Input: part model. Units: mm. Frame: model coordinates. Face numbers are marked on the shaded views. Give positions to 0.01 mm unless a question says otherwise; leave off trailing zeros. Loops run counter-clockwise (first coordinate to the right, second up) from the corner with the lowest first, then second, coordinate; pieces in that order, holes last. Notation, with made-up numbers: (52, 33) -> (56, 33) arc R29 cw to (56, 68) -> close; hole circle Ø9 at (72, 27). An arc over 180 degrees is marked (long way). Use CSV: the item, a comma, the result in double quotes.
```python
from build123d import *
from OCP.BRepFilletAPI import BRepFilletAPI_MakeChamfer

# Parameters (mm, degrees)
BOSS_EXTRUDE1_DEPTH  = 13.335
SKETCH2_R            = 13.97
BOSS_EXTRUDE2_DEPTH  = 2.54
BOSS_EXTRUDE3_DEPTH  = 36.068
BOSS_EXTRUDE4_START  = 6.477
SKETCH3_R            = 10.287
BOSS_EXTRUDE4_DEPTH  = 3.937
CHAMFER1_SIZE        = 0.254
CHAMFER1_EDGE_2_SIZE = 0.254
CHAMFER1_EDGE_3_SIZE = 0.254
CHAMFER1_EDGE_4_SIZE = 0.254
CHAMFER1_EDGE_5_SIZE = 0.254
CHAMFER1_EDGE_6_SIZE = 0.254
SKETCH4_W            = 12.192
SKETCH4_H            = 7.3025
CUT_EXTRUDE1_DEPTH   = 10.922
SKETCH5_W            = 6.35
SKETCH5_H            = 2.54
CUT_EXTRUDE2_DEPTH   = 6.35
SKETCH6_R            = 13.267076916
BOSS_EXTRUDE5_DEPTH  = 1.27
BOSS_EXTRUDE6_DEPTH  = 1.27
SKETCH8_R            = 2.54
BOSS_EXTRUDE7_DEPTH  = 2.54
FILLET1_R            = 1.27
SKETCH9_R            = 11.938
BOSS_EXTRUDE8_DEPTH  = 12.065
SKETCH10_R           = 13.97
BOSS_EXTRUDE9_DEPTH  = 2.54
SKETCH11_R           = 10.287
CUT_EXTRUDE3_DEPTH   = 6.223
SKETCH12_R           = 1.27
BOSS_EXTRUDE10_DEPTH = 9.525
CIRPATTERN1_COUNT    = 10
CHAMFER2_SIZE        = 1.27
CHAMFER2_SIZE2       = 0.733234842


with BuildPart() as part:
    # Sketch1 → Boss-Extrude1 (new body)
    with BuildSketch(Plane(origin=(0, 0, 0), x_dir=(1, 0, 0), z_dir=(0, 1, 0))):
        with BuildLine():
            Line((8.7122, -5.469912263), (8.7122, 5.469912263))
            ThreePointArc((8.7122, 5.469912263), (-10.287, 0), (8.7122, -5.469912263))
        make_face()
    extrude(amount=BOSS_EXTRUDE1_DEPTH)

    # Sketch2 → Boss-Extrude2 (add)
    with BuildSketch(Plane(origin=(0, 13.335, 0), x_dir=(1, 0, 0), z_dir=(0, 1, 0))):
        with Locations(Location((0, 0, 0), (0, 0, 270))):
            Circle(SKETCH2_R)
    extrude(amount=BOSS_EXTRUDE2_DEPTH)

    # Sketch1<2> → Boss-Extrude3 (add)
    with BuildSketch(Plane(origin=(0, 0, 0), x_dir=(1, 0, 0), z_dir=(0, 1, 0))):
        with BuildLine():
            Line((8.7122, -5.469912263), (8.7122, 5.469912263))
            ThreePointArc((8.7122, 5.469912263), (-10.287, 0), (8.7122, -5.469912263))
        make_face()
    extrude(amount=BOSS_EXTRUDE3_DEPTH)

    # Sketch3 → Boss-Extrude4 (add)
    with BuildSketch(Plane.XZ.offset(-13.335).offset(BOSS_EXTRUDE4_START)):
        Polygon((7.332348419, 12.7), (-7.332348419, 12.7), (-14.664696837, 0), (-7.332348419, -12.7), (7.332348419, -12.7), (14.664696837, 0), align=None)
        Circle(SKETCH3_R, mode=Mode.SUBTRACT)
    extrude(amount=-BOSS_EXTRUDE4_DEPTH)

    # Chamfer1
    chamfer1_edges = [part.edges().sort_by_distance(p)[0] for p in [
        (14.664696837, 8.8265, 0),
    ]]
    chamfer(chamfer1_edges, length=CHAMFER1_SIZE)

    # Chamfer1 edge 2
    chamfer1_edge_2_edges = [part.edges().sort_by_distance(p)[0] for p in [
        (7.332348419, 8.8265, 12.7),
    ]]
    chamfer(chamfer1_edge_2_edges, length=CHAMFER1_EDGE_2_SIZE)

    # Chamfer1 edge 3
    chamfer1_edge_3_edges = [part.edges().sort_by_distance(p)[0] for p in [
        (-7.332348419, 8.8265, 12.7),
    ]]
    chamfer(chamfer1_edge_3_edges, length=CHAMFER1_EDGE_3_SIZE)

    # Chamfer1 edge 4
    chamfer1_edge_4_edges = [part.edges().sort_by_distance(p)[0] for p in [
        (-14.664696837, 8.8265, 0),
    ]]
    chamfer(chamfer1_edge_4_edges, length=CHAMFER1_EDGE_4_SIZE)

    # Chamfer1 edge 5
    chamfer1_edge_5_edges = [part.edges().sort_by_distance(p)[0] for p in [
        (-7.332348419, 8.8265, -12.7),
    ]]
    chamfer(chamfer1_edge_5_edges, length=CHAMFER1_EDGE_5_SIZE)

    # Chamfer1 edge 6
    chamfer1_edge_6_edges = [part.edges().sort_by_distance(p)[0] for p in [
        (7.332348419, 8.8265, -12.7),
    ]]
    chamfer(chamfer1_edge_6_edges, length=CHAMFER1_EDGE_6_SIZE)

    # Sketch4 → Cut-Extrude1 (cut)
    with BuildSketch(Plane.XZ):
        Rectangle(SKETCH4_W, SKETCH4_H)
    cut_extrude1 = extrude(amount=-CUT_EXTRUDE1_DEPTH, mode=Mode.SUBTRACT)

    # Sketch5 → Cut-Extrude2 (cut)
    with BuildSketch(Plane.XZ):
        with Locations((0, -4.92125)):
            Rectangle(SKETCH5_W, SKETCH5_H)
    cut_extrude2 = extrude(amount=-CUT_EXTRUDE2_DEPTH, mode=Mode.SUBTRACT)

    # Mirror1: Cut-Extrude1, Cut-Extrude2 across plane
    add(cut_extrude1.mirror(Plane(origin=(0, 18.034, 0), x_dir=(0, 0, 1), z_dir=(0, -1, 0))), mode=Mode.SUBTRACT)
    add(cut_extrude2.mirror(Plane(origin=(0, 18.034, 0), x_dir=(0, 0, 1), z_dir=(0, -1, 0))), mode=Mode.SUBTRACT)

    # Sketch6 → Boss-Extrude5 (add)
    with BuildSketch(Plane.XZ.offset(-13.335)):
        with Locations(Location((0, 0, 0), (0, 0, 90))):
            Circle(SKETCH6_R)
    extrude(amount=BOSS_EXTRUDE5_DEPTH)

    # Sketch7 → Boss-Extrude6 (add)
    with BuildSketch(Plane.XZ.offset(-12.065)):
        with BuildLine():
            Line((-1.905, -10.109072361), (1.905, -10.109072361))
            Line((1.905, -10.109072361), (1.905, -86.309072361))
            ThreePointArc((1.905, -86.309072361), (0, -92.024072361), (-1.905, -86.309072361))
            Line((-1.905, -86.309072361), (-1.905, -10.109072361))
        make_face()
    extrude(amount=-BOSS_EXTRUDE6_DEPTH)

    # Sketch8 → Boss-Extrude7 (add)
    with BuildSketch(Plane(origin=(0, 13.335, 0), x_dir=(1, 0, 0), z_dir=(0, 1, 0))):
        with Locations(Location((0, 88.849072361, 0), (0, 0, 270))):
            Circle(SKETCH8_R)
    extrude(amount=BOSS_EXTRUDE7_DEPTH)

    # Fillet1
    fillet1_edges = [part.edges().sort_by_distance(p)[0] for p in [
        (0, 15.875, -91.389072361),
    ]]
    fillet(fillet1_edges, radius=FILLET1_R)

    # Sketch9 → Boss-Extrude8 (add)
    with BuildSketch(Plane.XZ.offset(-12.065)):
        with Locations(Location((0, -88.849072361, 0), (0, 0, 99.182197699))):
            Circle(SKETCH9_R)
    extrude(amount=BOSS_EXTRUDE8_DEPTH)

    # Sketch10 → Boss-Extrude9 (add)
    with BuildSketch(Plane.XZ):
        with Locations(Location((0, -88.849072361, 0), (0, 0, 270))):
            Circle(SKETCH10_R)
    extrude(amount=-BOSS_EXTRUDE9_DEPTH)

    # Sketch11 → Cut-Extrude3 (cut)
    with BuildSketch(Plane.XZ):
        with Locations(Location((0, -88.849072361, 0), (0, 0, 270))):
            Circle(SKETCH11_R)
    extrude(amount=-CUT_EXTRUDE3_DEPTH, mode=Mode.SUBTRACT)

    # Sketch12 → Boss-Extrude10 (add)
    with BuildSketch(Plane(origin=(0, 12.065, 0), x_dir=(1, 0, 0), z_dir=(0, 1, 0))):
        with Locations((0, 100.787072361)):
            Circle(SKETCH12_R)
    boss_extrude10 = extrude(amount=-BOSS_EXTRUDE10_DEPTH)

    # CirPattern1: Boss-Extrude10 ×10 about axis
    cirpattern1_axis = Axis((0, 0, -88.849072361), (0, 1, 0))
    for i in range(1, CIRPATTERN1_COUNT):
        add(boss_extrude10.rotate(cirpattern1_axis, i * 360 / CIRPATTERN1_COUNT))

    # Chamfer2: one chamfer whose edges measure the first distance from different faces: ONE call of the kernel's chamfer builder (chamfer() names one face for all edges)
    chamfer2_edges_1 = [part.edges().sort_by_distance(p)[0] for p in [
        (7.268848419, 6.858, -12.590014774),
    ]]
    chamfer2_side_1 = [part.faces().sort_by_distance(p)[0] for p in [
        (7.268848419, 8.8265, -12.590014774),
    ]]
    chamfer2_edges_2 = [part.edges().sort_by_distance(p)[0] for p in [
        (-7.268848419, 6.858, -12.590014774),
    ]]
    chamfer2_side_2 = [part.faces().sort_by_distance(p)[0] for p in [
        (-7.268848419, 8.8265, -12.590014774),
    ]]
    chamfer2_edges_3 = [part.edges().sort_by_distance(p)[0] for p in [
        (-14.537696837, 6.858, 0),
    ]]
    chamfer2_side_3 = [part.faces().sort_by_distance(p)[0] for p in [
        (-14.537696837, 8.8265, 0),
    ]]
    chamfer2_edges_4 = [part.edges().sort_by_distance(p)[0] for p in [
        (-7.268848419, 6.858, 12.590014774),
    ]]
    chamfer2_side_4 = [part.faces().sort_by_distance(p)[0] for p in [
        (-7.268848419, 8.8265, 12.590014774),
    ]]
    chamfer2_edges_5 = [part.edges().sort_by_distance(p)[0] for p in [
        (7.268848419, 6.858, 12.590014774),
    ]]
    chamfer2_side_5 = [part.faces().sort_by_distance(p)[0] for p in [
        (7.268848419, 8.8265, 12.590014774),
    ]]
    chamfer2_edges_6 = [part.edges().sort_by_distance(p)[0] for p in [
        (14.537696837, 6.858, 0),
    ]]
    chamfer2_side_6 = [part.faces().sort_by_distance(p)[0] for p in [
        (14.537696837, 8.8265, 0),
    ]]
    chamfer2 = BRepFilletAPI_MakeChamfer(part.part.solid().wrapped)
    for e in chamfer2_edges_1:
        chamfer2.Add(CHAMFER2_SIZE, CHAMFER2_SIZE2, e.wrapped, chamfer2_side_1[0].wrapped)  # the first distance lies on this face
    for e in chamfer2_edges_2:
        chamfer2.Add(CHAMFER2_SIZE, CHAMFER2_SIZE2, e.wrapped, chamfer2_side_2[0].wrapped)  # the first distance lies on this face
    for e in chamfer2_edges_3:
        chamfer2.Add(CHAMFER2_SIZE, CHAMFER2_SIZE2, e.wrapped, chamfer2_side_3[0].wrapped)  # the first distance lies on this face
    for e in chamfer2_edges_4:
        chamfer2.Add(CHAMFER2_SIZE, CHAMFER2_SIZE2, e.wrapped, chamfer2_side_4[0].wrapped)  # the first distance lies on this face
    for e in chamfer2_edges_5:
        chamfer2.Add(CHAMFER2_SIZE, CHAMFER2_SIZE2, e.wrapped, chamfer2_side_5[0].wrapped)  # the first distance lies on this face
    for e in chamfer2_edges_6:
        chamfer2.Add(CHAMFER2_SIZE, CHAMFER2_SIZE2, e.wrapped, chamfer2_side_6[0].wrapped)  # the first distance lies on this face
    add(Compound.cast(chamfer2.Shape()), mode=Mode.REPLACE)


solid = part.part
```
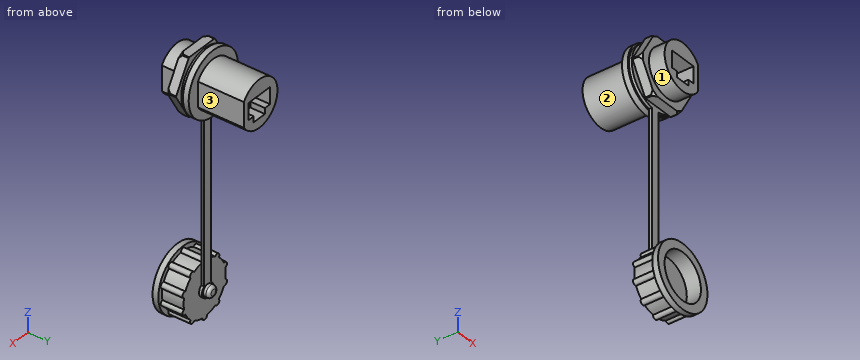
1) Section query B-B (z = -82). Return loops of the section in (x, y) (3 decimals), then the cut area to 3 significant figures.
From the geometry:
outline,"(-12.176, 0) -> (-7.675, 0) -> (-7.675, 6.223) -> (7.675, 6.223) -> (7.675, 0) -> (12.176, 0) -> (12.176, 2.54) -> (9.778, 2.54) -> (9.778, 12.065) -> (1.905, 12.065) -> (1.905, 13.335) -> (-1.905, 13.335) -> (-1.905, 12.065) -> (-9.778, 12.065) -> (-9.778, 2.54) -> (-12.176, 2.54) -> close"
area,"157 mm^2"
2) Mould query, pull axis Z, two halves, no side actions, for the marked faces 1, 2 and 3. Classes: pulls with the +Z half, pulls with the -Z half, needs draft (parallel to the pull), parting line crosses it, or undercut.
From the geometry:
face 1,"undercut"
face 2,"parting line crosses it"
face 3,"needs draft"
3) Section query A-A (y = 32). Return loops of the section in (x, z) (3 decimals), then the cut area to 3 significant figures.
From the geometry:
outline,"(8.712, -5.47) -> (8.712, 5.47) arc R10.287 ccw (long way) to start; hole (-6.096, -3.651) -> (-3.175, -3.651) -> (-3.175, -6.191) -> (3.175, -6.191) -> (3.175, -3.651) -> (6.096, -3.651) -> (6.096, 3.651) -> (-6.096, 3.651) -> close"
area,"216 mm^2"
4) Contact query for flat-ended pins moving along their axis: pin 1 (1 mm diameter, centred on y = 12.5, z = -46, fed in from +X) (3 decimals); pin 2 (6 mm diameter, centred on y = 33, z = -1, fed in from -X); pin 3 (2 mm diameter, centred on y = 28, z = 0.5, fed in from +X). Output: stop coordinate, or through.
From the geometry:
pin 1,"stops at x = 1.905"
pin 2,"stops at x = -10.29"
pin 3,"stops at x = 8.71"
5) Ray query, line 1 (Z direction, x = 2, y = 6); line 2 (Y direction, x = 0.5, z = -59.5) (3 decimals); line 3 (X direction, y = 5.5, z = -80). Return the intervals inside material, ascending.
From the geometry:
line 1,"z = -100.62 to -98.94, -78.76 to -77.08, -10.09 to -6.19, 3.65 to 10.09"
line 2,"y = 12.065 to 13.335"
line 3,"x = -8.01 to -5.25, 5.25 to 8.01"
